Could you check a few things on this model? Use its own coordinates, in mm. Face numbers are marked on the shaded views. A direction names the side the tool comes from. Give positions to 0.01 mm unless a question says otherwise; leave off trailing zeros. Write each loop counter-clockwise with the first axis right and the second up, starting at its lowest first coordinate (ties: lowest second). Pieces come first, ordered by that corner, then holes. Notation, with made-up numbers: M 70,63 L 123,63 A8 cw 123,76 Z; hole C 10.25,85 d9. An arc over 180 degrees is marked long. Answer as a JSON object with one key per item and string values. Group by question number.
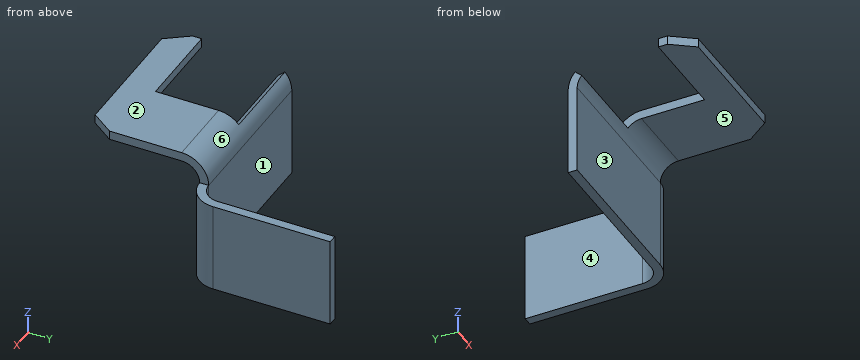
```python
from build123d import *

# Parameters (mm, degrees)
SM_BASE_FLANGE_1_DEPTH      = 10
SM_EDGE_FLANGE_2_DEPTH      = 18
SM_START                    = 1
SM_EDGE_FLANGE_2_FLAT_DEPTH = 1
SKETCH_10_W                 = 40
SKETCH_10_H                 = 40
CUT_EXTRUDE_1_DEPTH         = 29.460498942
SMNORMALCUT_DEPTH           = 10


# Read off the part's stored shape, not the designer's step: SMNormalCut
# Sheet-metal steps are written as plain solids
with BuildPart() as part:
    # Sketch 1 → 基体-法兰1 (new body)
    with BuildSketch(Plane.XY):
        with BuildLine():
            Line((0, 0), (18, 0))
            ThreePointArc((18, 0), (19.414213562, 0.585786438), (20, 2))
            Line((20, 2), (20, 15))
            Line((20, 15), (21, 15))
            Line((21, 15), (21, 2))
            ThreePointArc((21, 2), (20.121320344, -0.121320344), (18, -1))
            Line((18, -1), (0, -1))
            Line((0, -1), (0, 0))
        make_face()
    extrude(amount=SM_BASE_FLANGE_1_DEPTH)

    # 边线-法兰2 bend section (across the edge) → 边线-法兰2 (add)
    with BuildSketch(Plane(origin=(18, -1, 12), x_dir=(0, 0, -1), z_dir=(-1, 0, 0))):
        with BuildLine():
            Line((-1, 2), (0, 2))
            ThreePointArc((0, 2), (0.585786438, 0.585786438), (2, 0))
            Line((2, 0), (2, -1))
            ThreePointArc((2, -1), (-0.121320344, -0.121320344), (-1, 2))
        make_face()
    extrude(amount=SM_EDGE_FLANGE_2_DEPTH)

    # 边线-法兰2 profile (on flange) → 边线-法兰2 flat (add)
    with BuildSketch(Plane(origin=(0, -1, 12), x_dir=(-1, 0, 0), z_dir=(0, 0, 1)).offset(SM_START)):
        Polygon((0, 2), (0, 10), (-1.8, 12.5), (-16.2, 12.5), (-18, 10), (-18, 2), align=None)
    extrude(amount=-SM_EDGE_FLANGE_2_FLAT_DEPTH)

    # 草图10 → 切除-拉伸1 (cut, through all)
    with BuildSketch(Plane(origin=(0, 0, 12), x_dir=(-1, 0, 0), z_dir=(0, 0, -1))):
        with Locations((10, 10)):
            Rectangle(SKETCH_10_W, SKETCH_10_H)
    extrude(amount=-CUT_EXTRUDE_1_DEPTH, mode=Mode.SUBTRACT)

    # SMNormalCut outline → SMNormalCut (cut)
    with BuildSketch(Plane.YZ):
        with BuildLine():
            ThreePointArc((-3, 12), (-2.183503419, 11.825741858), (-1.509288015, 11.333333333))
            Line((-1.509288015, 11.333333333), (-0.763932023, 12))
            Line((-0.763932023, 12), (-3, 12))
        make_face()
    extrude(amount=SMNORMALCUT_DEPTH, mode=Mode.SUBTRACT)


solid = part.part
```
1) If we section it at A-A, the plane x = 2.75: List the corners of the cut face in (y, z) for me.
2) If we section it at D-D, the plane y = 4.25: List the corners of the cut face in (x, z) for me, plus the area to 3 significant figures.
3) If we section it at C-C, the plane x = 13.5: List the corners of the cut face in (y, z) for me.
4) I'm going to push flat-ended pins straight in: pin 1 (1.8 mm diameter, centred on y = -5.5, z = 12, fed in from -X); pin 2 (1.1 mm diameter, centred on x = 7, z = 12.5, fed in from +Y); pin 3 (1.5 mm diameter, centred on x = 18, z = 7.5, fed in from +Y). Where does each tip first touch, or does it pass through?
5) We'd pull the mould along Z, two halves only. Please class the marked faces 4, 5 and 6: released by +Z, released by -Z, zero draft, split by the parting line, or undercut.
6) Please list where these lines run through material, in increasing order: line 1 along Y through (x, z) = (10.75, 5.5); line 2 along Z through (x, y) = (2.25, -12); line 3 along X through (y, z) = (13.25, 1.5). Write a range as from..to.
7) If we section it at B-B, the plane z = 6.75: List the corners of the cut face in (x, y) for me.
8) For the marked faces 1, 2 and 3, which set-ups out of +Z, -Z, +X, -X, +Y, -Y let a thin tool reach every point of the face, with its end or its side?
Taken from the geometry:
{
 "1": {"outline": "M -13.5,12 L -10,12 L -10,13 L -13.5,13 Z; M -1.51,11.33 A2 cw -1,10 L -1,0 L 0,0 L 0,10 A3 ccw -0.76,12 Z"},
 "2": {"outline": "M 20,0 L 21,0 L 21,10 L 20,10 Z", "area": "10.0 mm²"},
 "3": {"outline": "M -13.5,12 L -3,12 A2 cw -1,10 L -1,0 L 0,0 L 0,10 A3 ccw -3,13 L -13.5,13 Z"},
 "4": {"pin 1": "x = 10", "pin 2": "y = -0.72", "pin 3": "y = 0.15"},
 "5": {"face 4": "zero draft", "face 5": "released by -Z", "face 6": "released by +Z"},
 "6": {"line 1": "-1..0", "line 2": "12..13", "line 3": "20..21"},
 "7": {"outline": "M 0,-1 L 18,-1 A3 ccw 21,2 L 21,15 L 20,15 L 20,2 A2 cw 18,0 L 0,0 Z"},
 "8": {"face 1": "+Z, -Z, -X, +Y", "face 2": "+Z, +X, -X, +Y, -Y", "face 3": "-Z, +X, -X, -Y"}
}
